For this review, take the finished solid that the model builds, in its own axes (mm). A direction names the side the tool comes from. Give positions to 0.01 mm unless a question says otherwise; leave off trailing zeros. Order: outer loops, then holes, each group sorted by start corner. A loop starts at its lowest first (then second) coordinate and runs counter-clockwise, first axis right, second up. Notation, with made-up numbers: (47.25, 44) -> (71.25, 44) arc R35 cw to (71.25, 76) -> close; hole circle Ø8 at (-10, 56). An arc over 180 degrees is marked (long way). Return JSON: item names as keys, results as strings. Group by question number.
1) To check wall thickness, follow line 1 along Z through (x, y) = (-20, 3.6); line 2 along Z through (x, y) = (-20, 0.8); line 3 along Z through (x, y) = (-100.11, 3). State the ranges of each line that lie inside material, in increasing order.
2) The part is to be moulded in two halves that separate along Z. For faces 1 (the face through (-58, 3, 100.75)), 2 (the face through (2, 7, 80)), 3 (the face through (-49.11, 1.01, 22.3)), say which applies: released by +Z, released by -Z, zero draft, split by the parting line, or undercut.
3) Insertion check: P1, Ø0.6, axis at y = 6, z = -0.5, coming from the +X side (3 decimals); P2, Ø1.1, axis at x = -117, y = 10, coming from the -Z side; P3, Ø1, axis at x = -75.5, z = -1, coming from the +Y side; P4, Ø1, axis at x = -90, y = 6, coming from the -Z side. Each pin has a flat end and moves straight along its axis. Give the tip position at first contact, or say it passes through.
4) Add section A-A (z = 6.72). Give the boundary of the cut face in (x, y).
5) For faces 4 (the face through (-48.7, 2, 76.4)), 5 (the face through (-117.74, 9.07, 74.1)), 6 (the face through (-116.73, 9, 78)), list the 3-axis set-ups (+Z, -Z, +X, -X, +Y, -Y) from which the entire face can be reached by the end or side of a thin tool; tool diameter is ignored.
6) Add section B-B (x = -20). Give the boundary of the cut face in (y, z), then the cut area to 3 significant figures.
7) Add section C-C (x = -6.58). Give the boundary of the cut face in (y, z), then the cut area to 3 significant figures.
8) Add section D-D (z = 30). Give the boundary of the cut face in (x, y).
Autodesk Inventor part; units mm, degrees
ref_plane "YZ Plane" through (0, 0, 0) normal (1, 0, 0) x (0, 1, 0)
ref_plane "XZ Plane" through (0, 0, 0) normal (0, 1, 0) x (-1, 0, 0)
ref_plane "XY Plane" through (0, 0, 0) normal (0, 0, 1) x (1, 0, 0)
sketch "Sketch1" plane through (0, 0, 0) normal (0, 1, 0) x (-1, 0, 0)
  line L0 (0, 0) -> (0, 98.75)
  line L1 (0, 98.75) -> (114.73, 98.75)
  line L2 (114.73, 98.75) -> (114.73, 0)
  line L3 (114.73, 0) -> (0, 0)
  line L4 (0, 98.75) -> (0, 90.47)
  circle A0 centre (11.7, 90.47) radius 1.65
  line L5 (0, 0) -> (0, 6.72)
  circle A1 centre (6.58, 6.72) radius 1.65
  line L6 (114.73, 0) -> (114.73, 9.87)
  circle A2 centre (100.11, 9.87) radius 1.65
  line L7 (-2, 0) -> (-2, 98.75)
  line L8 (-2, 98.75) -> (-2, 100.75)
  line L9 (-2, 100.75) -> (114.73, 100.75)
  line L10 (114.73, 100.75) -> (116.73, 100.75)
  line L11 (116.73, 100.75) -> (116.73, 0)
  line L12 (116.73, 0) -> (116.73, -2)
  line L13 (116.73, -2) -> (-2, -2)
  line L14 (-2, -2) -> (-2, 0)
  dimension "d11" = 2
  dimension "d12" = 2
  dimension "d13" = 2
  dimension "d14" = 2
extrude "Extrusion1" add sketch "Sketch1" along normal blind 4 contours L0 L1 L2 L3 | L7 L8 L9 L10 L11 L12 L13 L14
sketch "Sketch9" plane through (0, 4, 0) normal (0, 1, 0) x (1, 0, 0)
  circle A0 centre (-50, -75.0625) radius 1.65
  circle A1 centre (-20, -75.0625) radius 1.65
  circle A2 centre (-50, -23.6875) radius 1.65
  circle A3 centre (-20, -23.6875) radius 1.65
  point P0 (2, 2)
  dimension "d51" = 3.3
  dimension "d52" = 3.3
  dimension "d54" = 3.3
  dimension "d55" = 3.3
extrude "Extrusion9" cut sketch "Sketch9" against normal blind 10
sketch "Sketch10" plane through (0, 4, 0) normal (0, 1, 0) x (1, 0, 0)
  circle A0 centre (-50, -75.0625) radius 1.65
  circle A1 centre (-50, -75.0625) radius 3
  circle A2 centre (-50, -23.6875) radius 1.65
  circle A3 centre (-50, -23.6875) radius 3
  circle A4 centre (-20, -23.6875) radius 1.65
  circle A5 centre (-20, -23.6875) radius 3
  circle A6 centre (-20, -75.0625) radius 1.65
  circle A7 centre (-20, -75.0625) radius 3
  point P0 (0, 0)
  dimension "d58" = 6
  dimension "d59" = 6
  dimension "d60" = 6
  dimension "d61" = 6
extrude "Extrusion10" cut sketch "Sketch10" against normal blind 2
sketch "Sketch11" plane through (-116.73, 0, -2) normal (-1, 0, 0) x (0, 0, 1)
  line L0 (0, 0) -> (102.75, 0)
  line L1 (102.75, 4) -> (0, 4)
  line L2 (102.75, 0) -> (102.75, 4)
  line L3 (102.75, 4) -> (0, 4)
  line L4 (0, 0) -> (0, 4)
  line L5 (0, 4) -> (0, 0)
  line L6 (0, 0) -> (102.75, 0)
  point P0 (2, 0)
extrude "Extrusion11" add sketch "Sketch11" along normal blind 2
sketch "Sketch12" plane through (0, 4, 0) normal (0, 1, 0) x (1, 0, 0)
  line L0 (-118.73, -100.75) -> (-118.73, 2)
  line L1 (-118.73, -100.75) -> (-118.73, -80.75)
  line L2 (-118.73, -80.75) -> (-116.73, -80.75)
  line L3 (-116.73, -80.75) -> (-116.73, -70.75)
  line L4 (-116.73, -70.75) -> (-118.73, -70.75)
  line L5 (-118.73, -80.75) -> (-118.73, -70.75)
  line L6 (-118.73, 2) -> (-118.73, -18)
  line L7 (-118.73, -18) -> (-116.73, -18)
  line L8 (-116.73, -18) -> (-116.73, -28)
  line L9 (-116.73, -28) -> (-118.73, -28)
  line L10 (-118.73, -18) -> (-118.73, -28)
  point P0 (0, 0)
  dimension "d66" = 20
  dimension "d67" = 2
  dimension "d68" = 10
  dimension "d69" = 20
  dimension "d70" = 2
  dimension "d71" = 10
extrude "Extrusion12" add sketch "Sketch12" along normal blind 10
sketch "Sketch13" plane through (-118.73, 0, -2) normal (-1, 0, 0) x (0, 0, 1)
  line L0 (20, 14) -> (30, 14)
  line L1 (25, 14) -> (25, 9)
  line L2 (82.75, 14) -> (72.75, 14)
  line L3 (77.75, 14) -> (77.75, 9)
  circle A0 centre (25, 9) radius 1.65
  circle A1 centre (77.75, 9) radius 1.65
  point P0 (2, 0)
  dimension "d74" = 5
  dimension "d77" = 3.3
  dimension "d78" = 3.3
sketch "Sketch14" plane through (2, 0, 100.75) normal (1, 0, 0) x (0, 0, -1)
  line L0 (0, 4) -> (102.75, 4)
  line L1 (0, 0) -> (0, 4)
  line L2 (0, 4) -> (0, 0)
  line L3 (102.75, 0) -> (102.75, 4)
  line L4 (0, 0) -> (102.75, 0)
  line L5 (102.75, 0) -> (102.75, 4)
  line L6 (102.75, 4) -> (0, 4)
  point P0 (100.75, 0)
extrude "Extrusion13" add sketch "Sketch14" along normal blind 2
sketch "Sketch15" plane through (0, 4, 0) normal (0, 1, 0) x (1, 0, 0)
  line L0 (4, 2) -> (4, -100.75)
  line L1 (2, -49.375) -> (2, -44.375)
  line L2 (2, -44.375) -> (4, -44.375)
  line L3 (2, -49.375) -> (2, -54.375)
  line L4 (2, -54.375) -> (4, -54.375)
  line L5 (4, -44.375) -> (4, -44.7728)
  line L6 (4, -54.375) -> (4, -44.375)
  point P0 (0, 0)
  dimension "d82" = 5
  dimension "d83" = 5
extrude "Extrusion14" add sketch "Sketch15" along normal blind 10
sketch "Sketch16" plane through (4, 0, 100.75) normal (1, 0, 0) x (0, 0, -1)
  line L0 (56.375, 14) -> (46.375, 14)
  line L1 (51.375, 14) -> (51.375, 9)
  circle A0 centre (51.375, 9) radius 1.65
  point P0 (100.75, 0)
  dimension "d86" = 5
  dimension "d87" = 3.3
extrude "Extrusion15" cut sketch "Sketch16" against normal blind 10
extrude "Extrusion16" cut sketch "Sketch13" against normal blind 10
sketch "Sketch17" plane through (0, 4, 0) normal (0, 1, 0) x (1, 0, 0)
  line L0 (-71.73, 2) -> (-71.015, 2)
  line L1 (-71.015, 2) -> (-71.015, 0)
  line L2 (-71.015, 0) -> (-80.015, 0)
  line L3 (-80.015, 2) -> (-80.015, 0)
  line L4 (-80.015, 2) -> (-71.73, 2)
  line L5 (-118.73, 2) -> (4, 2)
  line L6 (-80.015, -100.75) -> (-80.015, -98.75)
  line L7 (-71.73, -98.75) -> (-71.015, -98.75)
  line L8 (-71.015, -98.75) -> (-71.015, -100.75)
  line L9 (-71.015, -100.75) -> (-80.015, -100.75)
  line L10 (-80.015, -98.75) -> (-71.73, -98.75)
  point P0 (0, 0)
  point P1 (-118.73, -100.75)
  dimension "d107" = 0.715
  dimension "d109" = 0.715
extrude "Extrusion17" add sketch "Sketch17" along normal blind 6
sketch "Sketch18" plane through (0, 4, 0) normal (0, 1, 0) x (1, 0, 0)
  line L0 (4, -54.375) -> (4, -100.75)
  line L1 (4, -100.75) -> (4, -86.75)
  line L2 (4, -86.75) -> (4, -72.75)
  line L3 (4, -72.75) -> (0, -72.75)
  line L4 (0, -72.75) -> (0, -86.75)
  line L5 (0, -86.75) -> (2, -86.75)
  line L6 (2, -86.75) -> (2, -72.75)
  point P0 (0, 0)
  dimension "d100" = 14
  dimension "d101" = 14
  dimension "d102" = 4
  dimension "d103" = 2
extrude "Extrusion18" add sketch "Sketch18" along normal blind 6
fillet "Fillet1" radius 1 9 edges at (4, 14, 49.375) (4, 9, 44.375) (4, 9, 54.375) (4, 4, 21.1875) (-118.73, 9, 80.75) (-118.73, 14, 75.75) (-118.73, 9, 70.75) (-118.73, 14, 23) (-118.73, 9, 18)
fillet "Fillet2" radius 1 2 edges at (-118.4371, 13.7071, 28) (-118.73, 8.5, 28)
properties part number "case"
Evaluation:
{
 "1": {"line 1": "-2 to 20.69, 26.69 to 72.06, 78.06 to 100.75", "line 2": "-2 to 22.04, 25.34 to 73.41, 76.71 to 100.75", "line 3": "-2 to 8.22, 11.52 to 100.75"},
 "2": {"face 1": "released by +Z", "face 2": "zero draft", "face 3": "undercut"},
 "3": {"P1": "x = -71.015", "P2": "z = 18", "P3": "y = 10", "P4": "through"},
 "4": {"outline": "(-118.73, 0) -> (-8.23, 0) -> (-8.23, 4) -> (-118.73, 4) -> close; (-4.93, 0) -> (4, 0) -> (4, 3) arc R1 ccw to (3, 4) -> (-4.93, 4) -> close"},
 "5": {"face 4": "+Y", "face 5": "-X", "face 6": "+Z, -Z, +Y"},
 "6": {"outline": "(0, -2) -> (4, -2) -> (4, 20.69) -> (2, 20.69) -> (2, 22.04) -> (0, 22.04) -> close; (0, 25.34) -> (2, 25.34) -> (2, 26.69) -> (4, 26.69) -> (4, 72.06) -> (2, 72.06) -> (2, 73.41) -> (0, 73.41) -> close; (0, 76.71) -> (2, 76.71) -> (2, 78.06) -> (4, 78.06) -> (4, 100.75) -> (0, 100.75) -> close", "area": "374 mm^2"},
 "7": {"outline": "(0, -2) -> (4, -2) -> (4, 5.07) -> (0, 5.07) -> close; (0, 8.37) -> (4, 8.37) -> (4, 100.75) -> (0, 100.75) -> close", "area": "398 mm^2"},
 "8": {"outline": "(-118.73, 0) -> (4, 0) -> (4, 3) arc R1 ccw to (3, 4) -> (-118.73, 4) -> close"}
}
